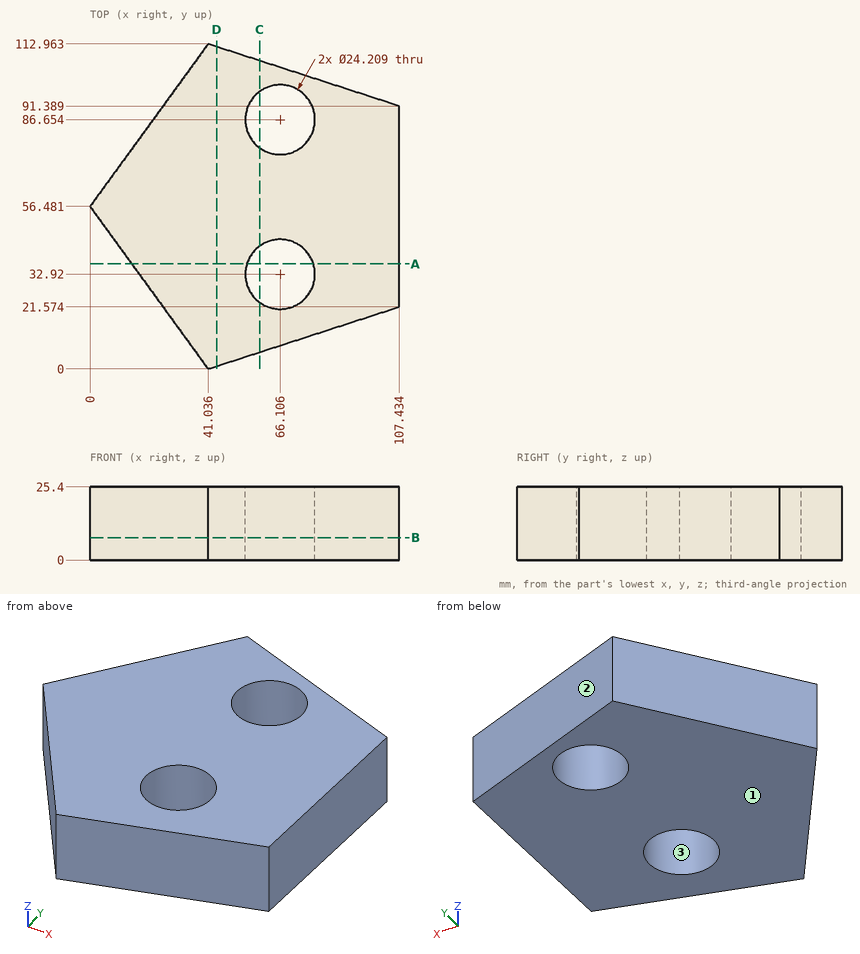
Source: three-view drawing plus pictorial views. Frame: mm from the lowest corner of the part. Coordinates: 2 decimals unless noted, no trailing zeros. Order: outer loops, then holes, each group sorted by start corner. A loop starts at its lowest first (then second) coordinate and runs counter-clockwise, first axis right, second up.
Item 1: Cut plane B-B (z = 7.75). Return loops of the section in (x, y) (1 decimal).
Output values:
outline: (0, 56.5) - (41, 0) - (107.4, 21.6) - (107.4, 91.4) - (41, 113) - close; hole circle Ø24.2 at (66.1, 32.9); hole circle Ø24.2 at (66.1, 86.7)
Item 2: First-contact query: P1, Ø4, axis at y = 100.5, z = 22, coming from the -X side; P2, Ø10, axis at x = 29, z = 12, coming from the -Y side (1 decimal); P3, Ø1.5, axis at x = 91.5, z = 17, coming from the +Y side. Flat tips, straight axial feed; report the tip coordinate or a pass-through.
Output values:
P1: stops at x = 30.53
P2: stops at y = 9.7
P3: stops at y = 96.81
Item 3: Material intervals for line 1 (Y direction, x = 61, z = 24.25) (1 decimal); line 2 (Y direction, x = 72.5, z = 18) (1 decimal); line 3 (X direction, y = 77, z = 15.5) (1 decimal), sorted ascending.
Output values:
line 1: y = 6.5 to 21.9, 43.9 to 75.7, 97.6 to 106.5
line 2: y = 10.2 to 22.6, 43.2 to 76.4, 96.9 to 102.7
line 3: x = 14.9 to 58.8, 73.4 to 107.4
Item 4: Cut plane D-D (x = 44). Return loops of the section in (y, z), plus the area to 3 significant figures.
Output values:
outline: (0.96, 0) - (112, 0) - (112, 25.4) - (0.96, 25.4) - close
area: 2,820 mm2
Item 5: Cut plane C-C (x = 59). Return loops of the section in (y, z) (1 decimal).
Output values:
outline: (5.8, 0) - (23.1, 0) - (23.1, 25.4) - (5.8, 25.4) - close; (42.7, 0) - (76.9, 0) - (76.9, 25.4) - (42.7, 25.4) - close; (96.5, 0) - (107.1, 0) - (107.1, 25.4) - (96.5, 25.4) - close
Item 6: Cut plane A-A (y = 36.5). Return loops of the section in (x, z), plus the area to 3 significant figures.
Output values:
outline: (14.52, 0) - (54.54, 0) - (54.54, 25.4) - (14.52, 25.4) - close; (77.67, 0) - (107.43, 0) - (107.43, 25.4) - (77.67, 25.4) - close
area: 1,770 mm2
Item 7: Pull-direction query (Y, two-part tool) for the marked faces 1, 2 and 3; classes: pulls with the +Y half, pulls with the -Y half, needs draft (parallel to the pull), parting line crosses it, or undercut.
Output values:
face 1: needs draft
face 2: pulls with the +Y half
face 3: undercut
